Can you work these out from the model? Positions are in its coordinate system, mm. Face numbers are marked on the shaded views. A direction names the side the tool comes from. Round coordinates to 2 decimals unless told otherwise and drop trailing zeros. Order: outer loops, then holes, each group sorted by start corner. A loop starts at its lowest first (then second) coordinate and runs counter-clockwise, first axis right, second up.
Q1. For the marked faces 1 and 2, which set-ups out of +Z, -Z, +X, -X, +Y, -Y let a thin tool reach every point of the face, with its end or its side?
Q2. Will these pins go through, and if not, where does the flat tip stop? P1, Ø1.5, axis at y = 0.5, z = -4.5, coming from the +X side; P2, Ø1.5, axis at x = -0.5, z = 13, coming from the -Y side.
Q3. If we section it at B-B (z = -3.25): Please give me the cut outline in (x, y), plus the area to 3 significant figures.
Q4. If I drill on line 1 (Y direction, x = -0.15, z = 3.75); line 2 (Z direction, x = -1.5, y = 1.15); line 3 (X direction, y = -2, z = 12.75), over which ranges is the centre line in solid material (lowest first)?
Q5. If we section it at A-A (z = 12.5): Please give me the cut outline in (x, y), plus the area to 3 significant figures.
from build123d import *

# Parameters (mm, degrees)
F0_W     = 8.9162653312
F0_H     = 68.7855742872
F5_R     = 0.2551301714
F3_R     = 0.2579924581
F7_SCALE = 0.2717


with BuildPart() as f1:
    # F0 (on Front) → F1 (revolve)
    with BuildSketch(Plane.XZ):
        Polygon((0, 42.8588315845), (0, 40.7245121896), (8.9162653312, 40.7245121896), (10.7394016028, 54.0099740028), (9.4826271558, 49.960937351), (9.3766475536, 49.6194955792), (7.2782151401, 42.8588315845), (2.2957634175, 42.8588315845), align=None)
        with Locations((4.4581326656, 6.331725046)):
            Rectangle(F0_W, F0_H)
    revolve(axis=Axis((0, 0, 41.791671887), (0, 0, -1)))

    # F5 (on offset) → F6 section 0
    with BuildSketch(Plane.XY.offset(42.8498)):
        Circle(F5_R)
    # F3 (on offset) → F6 section 1
    with BuildSketch(Plane.XY.offset(65.024)):
        Circle(F3_R)
    loft()


with BuildPart() as f1_1:
    # F7: moved
    add(f1.part.scale(F7_SCALE))


solid = f1_1.part
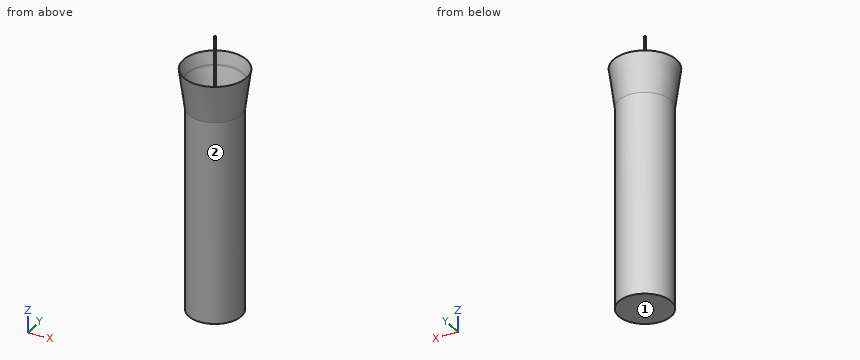
Solution:
1. face 1: -Z, +X, -X, +Y, -Y
1. face 2: -Z
2. P1: stops at x = 2.42
2. P2: stops at y = -2.78
3. outline: circle Ø4.85 at (0, 0)
3. area: 18.4 mm2
4. line 1: y = -2.42 to 2.42
4. line 2: z = -7.62 to 11.64
4. line 3: x = -1.74 to -1.18, 1.18 to 1.74
5. outline: circle Ø5.24 at (0, 0); circle Ø0.14 at (0, 0); hole circle Ø4.49 at (0, 0)
5. area: 5.77 mm2
